from build123d import *

# Parameters (mm, degrees)
F0_W     = 116.6634205729
F0_H     = 76.1592537165
F0_W_2   = 60.1857760921
F0_H_2   = 5.1343319938
F1_DEPTH = 25.4
F2_W     = 46.4942213148
F2_H     = 6.5605351701
F3_DEPTH = 25.4
F4_T     = -2.54


with BuildPart() as f1:
    # F0 (on Front) → F1 (new body)
    with BuildSketch(Plane.XZ):
        with Locations((27.2404802963, -5.7048127055)):
            Rectangle(F0_W, F0_H)
        with Locations((19.8242249899, 15.8308562823)):
            Rectangle(F0_W_2, F0_H_2, mode=Mode.SUBTRACT)
    extrude(amount=F1_DEPTH)

    # F2 (on face) → F3 (join)
    with BuildSketch(Plane.XZ.offset(25.4)):
        with Locations((37.3461479321, -16.8291977607)):
            Rectangle(F2_W, F2_H)
    extrude(amount=F3_DEPTH)

    # F4
    f4_openings = [f1.faces().sort_by_distance(p)[0] for p in [
        (37.346148, -50.8, -16.829198),
    ]]
    offset(amount=F4_T, openings=f4_openings, kind=Kind.INTERSECTION)


solid = f1.part
Part model, mm, in its own coordinate system. A direction names the side the tool comes from. Coordinates: 2 decimals unless noted, no trailing zeros. Loops run counter-clockwise (first coordinate to the right, second up) from the corner with the lowest first, then second, coordinate; pieces in that order, holes last. Notation, with made-up numbers: M 79.25,-1.75 L 116.25,-1.75 A14 cw 116.25,20.25 Z; hole C 88,39.25 d11. An arc over 180 degrees is marked long. Use a Markdown table: item, result. Add a question column.
Q1. Probe L1, parallel to Z at x = -4, y = -10; L2, parallel to Y at x = -21, z = 16.5; L3, parallel to X at y = -14.5, z = 24.5. List the from-to ranges inside material, lowest first.
Q2. Which spindle directions (+Z, -Z, +X, -X, +Y, -Y) get a long thin tool onto all of the face, cutting with end or side? Do faces 1 (the flat face through (26, -13, 29.835)), 2 (the flat face through (37, -38, -20.109)), 3 (the flat face through (37, -37, -16.089)), 4 (the flat face through (19, -13, 13.264)). Say none if no direction does.
Q3. Cut at D-D (z = -12). Write the cut outline in (x, y), and give its area (3 significant figures).
Q4. Mould opens along Y. For faces 5 (the flat face through (49.917, -13, 16)), 6 (the flat face through (26, -2.54, -5)), 7 (the flat face through (-12.809, -13, 16)), 8 (the flat face through (26, 0, -5)) say: +Y half, -Y half, draft (parallel to the pull), parting line (faces both ways), or undercut.
Q5. Cut at C-C (y = -30). Write the cut outline in (x, z), and give its area (3 significant figures).
Q6. Pin check, flat tips, straight feed: P1, Ø7, axis at y = -35, z = -17.5, coming from the +X side; P2, Ø6, axis at x = 39.5, z = 24.5, coming from the -Y side; P3, Ø2, axis at x = 15, y = -31.5, coming from the -Z side. Stop position of each tip, or through.
Q7. Cut at A-A (y = -12). Write the cut outline in (x, z).
Q8. Cut at B-B (x = 42). Write the cut outline in (y, z), and give its area (3 significant figures).
Worked out:
| question | item | result |
|---|---|---|
| 1 | L1 | z = -43.78 to -41.24, 10.72 to 13.26, 18.4 to 20.94, 29.83 to 32.37 |
| 1 | L2 | y = -25.4 to -22.86, -2.54 to 0 |
| 1 | L3 | x = -31.09 to -28.55, 83.03 to 85.57 |
| 2 | face 1 | none |
| 2 | face 2 | -Z, +X, -X, -Y |
| 2 | face 3 | -Y |
| 2 | face 4 | +Y, -Y |
| 3 | outline | M -31.09,-25.4 L 85.57,-25.4 L 85.57,0 L -31.09,0 Z; hole M -28.55,-22.86 L 83.03,-22.86 L 83.03,-2.54 L -28.55,-2.54 Z |
| 3 | area | 696 mm2 |
| 4 | face 5 | draft |
| 4 | face 6 | undercut |
| 4 | face 7 | undercut |
| 4 | face 8 | +Y half |
| 5 | outline | M 14.1,-20.11 L 60.59,-20.11 L 60.59,-13.55 L 14.1,-13.55 Z; hole M 16.64,-17.57 L 58.05,-17.57 L 58.05,-16.09 L 16.64,-16.09 Z |
| 5 | area | 244 mm2 |
| 6 | P1 | stops at x = 60.59 |
| 6 | P2 | stops at y = -25.4 |
| 6 | P3 | stops at z = -20.11 |
| 7 | outline | M -31.09,-43.78 L 85.57,-43.78 L 85.57,32.37 L -31.09,32.37 Z; M -12.81,10.72 L 52.46,10.72 L 52.46,20.94 L -12.81,20.94 Z; hole M -28.55,-41.24 L 83.03,-41.24 L 83.03,29.83 L -28.55,29.83 Z; hole M -10.27,13.26 L 49.92,13.26 L 49.92,18.4 L -10.27,18.4 Z |
| 8 | outline | M -50.8,-20.11 L -25.4,-20.11 L -25.4,-43.78 L 0,-43.78 L 0,13.26 L -25.4,13.26 L -25.4,-13.55 L -50.8,-13.55 L -50.8,-16.09 L -22.86,-16.09 L -22.86,10.72 L -2.54,10.72 L -2.54,-41.24 L -22.86,-41.24 L -22.86,-17.57 L -50.8,-17.57 Z; M -25.4,18.4 L 0,18.4 L 0,32.37 L -25.4,32.37 Z; hole M -22.86,20.94 L -2.54,20.94 L -2.54,29.83 L -22.86,29.83 Z |
| 8 | area | 693 mm2 |
